Check sheet for the modelled part. Datum: model origin and axes. Units: mm. Face numbers are marked on the shaded views. A direction names the side the tool comes from. Round coordinates to 2 decimals unless told otherwise and drop trailing zeros. Write each loop counter-clockwise with the first axis right and the second up, starting at its lowest first coordinate (ties: lowest second). Pieces come first, ordered by that corner, then holes.
Item 1: Tool access check on the marked faces 1, 2, 3, 4 and 5. Record the directions out of +Z, -Z, +X, -X, +Y, -Y that give a thin tool (end or side, any length) a straight path to the whole face; none if there is none.
Item 2: Material ranges on line 1 (Y direction, x = 0, z = 17); line 2 (X direction, y = -33.5, z = 16.25); line 3 (Z direction, x = -15.5, y = -22.75), recorded low to high.
Item 3: Go/stop test with flat-tipped pins: pin 1 Ø1.5 at (y, z) = (-36, 20.5) entering from -X (3 decimals); pin 2 Ø1.5 at (x, z) = (-14.5, 17) entering from -Y; pin 3 Ø12 at (x, z) = (6, 17) entering from +Y; pin 4 Ø5 at (x, z) = (4, 15.5) entering from -Y. Record where each tip stops, or that it passes through.
Item 4: Cross-section at A-A on x = 0. Enter the section's corners in (y, z), plus the area to 4 significant figures.
Item 5: Cross-section at B-B on x = -6.5. Enter the section's corners in (y, z), plus the area to 3 significant figures.
Item 6: Release check for a two-part mould opening along Y. For the marked faces 6, 7 and 8 record: +Y half, -Y half, draft (parallel to the pull), parting line (faces both ways), or undercut.
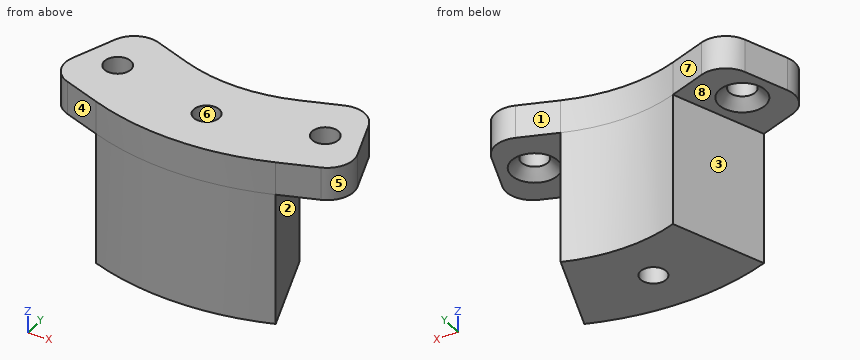
Autodesk Inventor part; units mm, degrees
ref_plane "YZ Plane" through (0, 0, 0) normal (1, 0, 0) x (0, 1, 0)
ref_plane "XZ Plane" through (0, 0, 0) normal (0, 1, 0) x (-1, 0, 0)
ref_plane "XY Plane" through (0, 0, 0) normal (0, 0, 1) x (1, 0, 0)
sketch "Sketch1" plane through (0, 0, 0) normal (0, 0, 1) x (1, 0, 0)
  circle A0 centre (0, 0) radius 40
  circle A1 centre (0, 0) radius 32.5
  circle A2 centre (0, 0) radius 25
  line L0 (-8.5505, -23.4923) -> (-13.6808, -37.5877)
  line L1 (0, 0) -> (57.2098, 0) construction
  line L2 (8.5505, -23.4923) -> (13.6808, -37.5877)
  line L3 (0, 0) -> (61.497, 0) construction
  point P0 (0, -32.5)
  dimension "d1" = 65
  dimension "d0" = 80
  dimension "d2" = 50
  dimension "d4" = 110
  dimension "d6" = 70
extrude "Extrusion1" add sketch "Sketch1" along normal blind 20 contours L0 A1 L2 A0 | L0 A2 L2 A1 picked at (0, -34.8535) picked at (-0.9674, -29.7972)
sketch "Sketch2" plane through (0, 0, 20) normal (0, 0, 1) x (1, 0, 0)
  arc A0 (-13.6808, -37.5877) -> (13.6808, -37.5877) centre (0, 0) ccw
  line L0 (13.6808, -37.5877) -> (8.5505, -23.4923)
  arc A1 (-8.5505, -23.4923) -> (8.5505, -23.4923) centre (0, 0) ccw
  line L1 (-8.5505, -23.4923) -> (-13.6808, -37.5877)
  line L2 (8.5505, -23.4923) -> (17.9474, -20.0721)
  line L3 (17.9474, -20.0721) -> (23.0777, -34.1675)
  line L4 (23.0777, -34.1675) -> (13.6808, -37.5877)
  line L5 (-13.6808, -37.5877) -> (-23.0777, -34.1675)
  line L6 (-23.0777, -34.1675) -> (-17.9474, -20.0721)
  line L7 (-8.5505, -23.4923) -> (-13.6808, -37.5877)
  line L8 (-17.9474, -20.0721) -> (-8.5505, -23.4923)
  circle A2 centre (15.8141, -28.8299) radius 2
  circle A3 centre (-15.8141, -28.8299) radius 2
  dimension "d9" = 10
  dimension "d10" = 10
  dimension "d11" = 4
  dimension "d12" = 4
  dimension "d13" = 7.5
  dimension "d14" = 7.5
  dimension "d15" = 5
  dimension "d16" = 5
extrude "Extrusion2" add sketch "Sketch2" along normal blind 5
chamfer "Chamfer1" distance 1.5 angle 45 2 edges at (-17.8141, -28.8299, 20) (13.8141, -28.8299, 20)
fillet "Fillet1" radius 4 4 edges at (17.9474, -20.0721, 22.5) (-17.9474, -20.0721, 22.5) (-23.0777, -34.1675, 22.5) (23.0777, -34.1675, 22.5)
hole "Hole1" at (0, -32.5, 0) direction (0, 0, 1) diameter 3.9 end through all
equation "\"d10\" = d9"
properties part number "3DP_ABS_Bowl_Feeder_Standoff" material "ABS Plastic"
Response values:
1. face 1: +Z, -Z, +Y
1. face 2: -Z, +X, +Y
1. face 3: -Z, -X, +Y
1. face 4: +Z, -Z, -X, -Y
1. face 5: +Z, -Z, +X
2. line 1: y = -40 to -34.45, -30.55 to -25
2. line 2: x = -12.19 to -1.67, 1.67 to 12.19
2. line 3: z = 20 to 25
3. pin 1: stops at x = -19.935
3. pin 2: passes through
3. pin 3: stops at y = -22.53
3. pin 4: stops at y = -39.97
4. outline: (-40, 0) - (-34.45, 0) - (-34.45, 25) - (-40, 25) - close; (-30.55, 0) - (-25, 0) - (-25, 25) - (-30.55, 25) - close
4. area: 277.5 mm2
5. outline: (-39.47, 0) - (-24.14, 0) - (-24.14, 25) - (-39.47, 25) - close
5. area: 383 mm2
6. face 6: undercut
6. face 7: +Y half
6. face 8: draft
